For this review, take the finished solid that the model builds, in its own axes (mm). Coordinates: 2 decimals unless noted, no trailing zeros. Loops run counter-clockwise (first coordinate to the right, second up) from the corner with the lowest first, then second, coordinate; pieces in that order, holes last.
1. Take a section at A-A, the plane z = 15.5. State the section outline as (x, y) points.
2. To check wall thickness, follow probe 1 along X at (y, z) = (-16.5, 6.75); probe 2 along Y at (x, z) = (-2.5, 20.25); probe 3 along X at (y, z) = (-10, 9.5). State the ranges of each line that lie inside material, in increasing order.
3. Clearance check with a flat-ended pin moving along its axis: P1, Ø12, axis at y = -18.5, z = 6, coming from the +X side. State where the tip first meets the part, or that it passes through.
```python
from build123d import *

# Parameters (mm, degrees)
F1_DEPTH = 25.4
F2_R     = 5.08
F3_SIZE  = 5.08


with BuildPart() as f1:
    # F0 (on Top) → F1 (new body)
    with BuildSketch(Plane.XY):
        with BuildLine():
            ThreePointArc((0, -21.4998775326), (-15.202709198, -15.202709198), (-21.4998775326, 0))
            Line((-21.4998775326, 0), (-57.4172474444, 0))
            Line((-57.4172474444, 0), (-57.4172474444, -38.9976762235))
            Line((-57.4172474444, -38.9976762235), (0, -38.9976762235))
            Line((0, -38.9976762235), (0, -21.4998775326))
        make_face()
    extrude(amount=F1_DEPTH)

    # F2
    f2_edges = [f1.edges().sort_by_distance(p)[0] for p in [
        (-28.708624, -38.997676, 25.4),
    ]]
    fillet(f2_edges, radius=F2_R)

    # F3
    f3_edges = [f1.edges().sort_by_distance(p)[0] for p in [
        (-15.202709, -15.202709, 25.4),
    ]]
    chamfer(f3_edges, length=F3_SIZE)


solid = f1.part
```
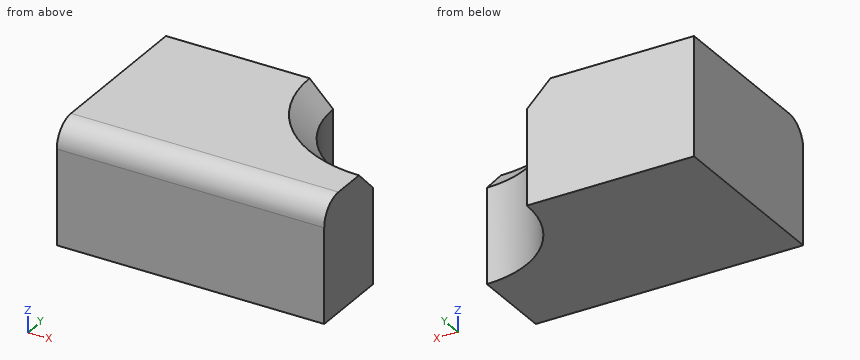
Results list:
1. outline: (-57.42, -39) - (0, -39) - (0, -21.5) arc R21.5 cw to (-21.5, 0) - (-57.42, 0) - close
2. probe 1: x = -57.42 to -13.78
2. probe 2: y = -39 to -21.35
2. probe 3: x = -57.42 to -19.03
3. P1: stops at x = 0
